Here's how the part is built. I have some questions about the finished solid (model axes, mm). Face numbers are marked on the shaded views. Give positions to 0.01 mm unless a question says otherwise; leave off trailing zeros. Loops run counter-clockwise (first coordinate to the right, second up) from the corner with the lowest first, then second, coordinate; pieces in that order, holes last. Notation, with made-up numbers: (-34.75, 73) - (-22.75, 73) arc R6 ccw to (-22.75, 82) - close; hole circle Ø8 at (37.5, 68.25). An arc over 180 degrees is marked (long way). Return JSON: item names as keys, results as strings. Group by question number.
(1) I need wall thicknesses on probe 1 along Z at (x, y) = (-36, 1.75); probe 2 along X at (y, z) = (3.25, 2); probe 3 along X at (y, z) = (3, 15). Which ranges of each line are inside material? Lowest first, please. Write a range as [from, to].
(2) For P1, Ø1, axis at x = -33.5, y = 5, coming from the +Z side (3 decimals); P2, Ø2, axis at x = 22.5, y = 1, coming from the -Z side; P3, Ø13, axis at x = 34.925, z = 15.875, coming from the +Y side; P4, Ø3, axis at y = 5.5, z = -11, coming from the +X side, each with a flat end and sliding along its axis, tell me the tip position at first contact or that it passes through.
(3) If we section it at C-C (y = 3): State how many separate pieces and enclosed holes the cut face has, then the cut area to 3 significant figures.
(4) If we section it at A-A (x = 0): Please give me the cut outline in (y, z), then the cut area to 3 significant figures.
(5) If we mould it in two halves opening along X, with no side actions, what happens to the marked faces 1, 2, 3 and 4? For each: released by +X, released by -X, zero draft, split by the parting line, or undercut.
(6) If we section it at D-D (z = 3): Please give me the cut outline in (x, y).
(7) If we section it at B-B (z = 13): Please give me the cut outline in (x, y).
```python
from build123d import *

# Parameters (mm, degrees)
SKETCH1_R               = 14.2875
BOSS_EXTRUDE1_DEPTH     = 6.35
F_3_8_CLEARANCE_HOLE1_D = 10.0838


with BuildPart() as part:
    # Sketch1 → Boss-Extrude1 (new body)
    with BuildSketch(Plane(origin=(0, 0, 0), x_dir=(1, 0, 0), z_dir=(0, 1, 0))):
        with BuildLine():
            Line((-41.209227539, -8.717199414), (-13.615826335, 15.508567937))
            ThreePointArc((-13.615826335, 15.508567937), (0, 20.6375), (13.615826335, 15.508567937))
            Line((13.615826335, 15.508567937), (41.209227539, -8.717199414))
            ThreePointArc((41.209227539, -8.717199414), (43.636188178, -19.727379203), (33.858044807, -25.340053176))
            ThreePointArc((33.858044807, -25.340053176), (0, -23.437740611), (-33.858044807, -25.340053176))
            ThreePointArc((-33.858044807, -25.340053176), (-43.636188178, -19.727379203), (-41.209227539, -8.717199414))
        make_face()
        with Locations(Location((0, 0, 0), (0, 0, 270))):
            Circle(SKETCH1_R, mode=Mode.SUBTRACT)
    extrude(amount=BOSS_EXTRUDE1_DEPTH)

    # 3/8 Clearance Hole1 (through all)
    with Locations(Plane(origin=(0, 6.35, 0), x_dir=(1, 0, 0), z_dir=(0, 1, 0))):
        with Locations((-34.925, -15.875), (34.925, -15.875)):
            Hole(F_3_8_CLEARANCE_HOLE1_D / 2)


solid = part.part
```
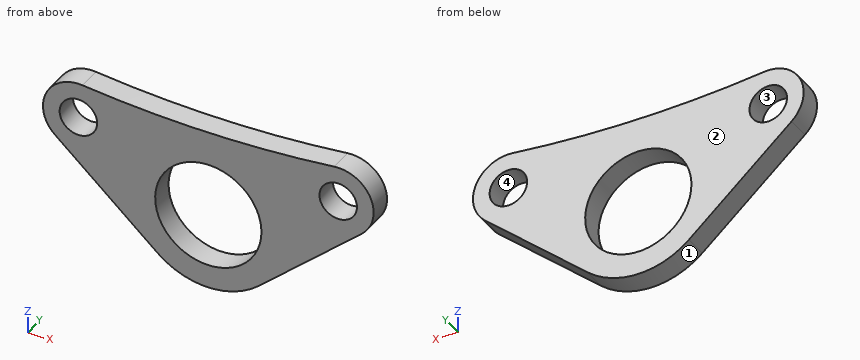
Values:
{
 "1": {"probe 1": "[4.14, 10.95], [20.8, 25.34]", "probe 2": "[-33.56, -14.15], [14.15, 33.56]", "probe 3": "[-44.41, -39.89], [-29.96, 29.96], [39.89, 44.41]"},
 "2": {"P1": "z = 25.355", "P2": "z = -8.59", "P3": "y = 6.35", "P4": "x = 20.46"},
 "3": {"separate pieces": "1", "enclosed holes": "3", "area": "1,960 mm2"},
 "4": {"outline": "(0, -20.64) - (6.35, -20.64) - (6.35, -14.29) - (0, -14.29) - close; (0, 14.29) - (6.35, 14.29) - (6.35, 23.44) - (0, 23.44) - close", "area": "98.4 mm2"},
 "5": {"face 1": "split by the parting line", "face 2": "zero draft", "face 3": "undercut", "face 4": "undercut"},
 "6": {"outline": "(-34.7, 0) - (-13.97, 0) - (-13.97, 6.35) - (-34.7, 6.35) - close; (13.97, 0) - (34.7, 0) - (34.7, 6.35) - (13.97, 6.35) - close"},
 "7": {"outline": "(-44.01, 0) - (-39.07, 0) - (-39.07, 6.35) - (-44.01, 6.35) - close; (-30.78, 0) - (-5.93, 0) - (-5.93, 6.35) - (-30.78, 6.35) - close; (5.93, 0) - (30.78, 0) - (30.78, 6.35) - (5.93, 6.35) - close; (39.07, 0) - (44.01, 0) - (44.01, 6.35) - (39.07, 6.35) - close"}
}
